Source: CAD feature listing. Evaluate the final solid. Frame: model axes, mm. Coordinates: 2 decimals unless noted, no trailing zeros. Write each loop counter-clockwise with the first axis right and the second up, starting at its lowest first coordinate (ties: lowest second). Pieces come first, ordered by that corner, then holes. Notation, with made-up numbers: (17, 47) -> (30, 47) arc R26 ccw to (30, 66) -> close; hole circle Ø6 at (62.5, 78.25). An arc over 180 degrees is marked (long way). Write item = value, one per line.
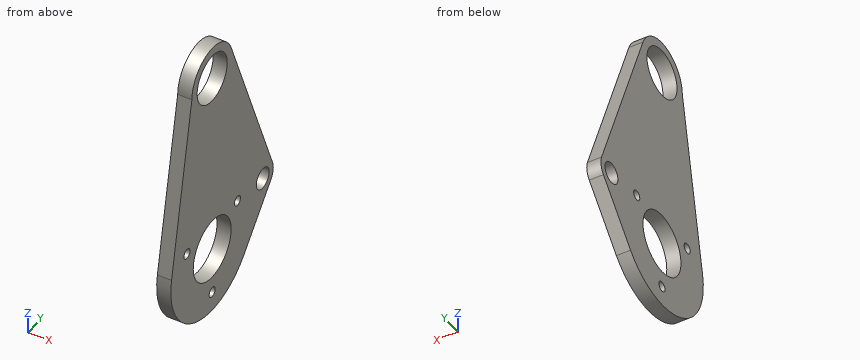
from build123d import *

# Parameters (mm, degrees)
SKETCH1_R            = 11.1125
SKETCH1_R_2          = 14
SKETCH1_R_3          = 4.7625
BOSS_EXTRUDE1_DEPTH  = 3.175
M4_CLEARANCE_HOLE1_D = 4.5


with BuildPart() as part:
    # Sketch1 → Boss-Extrude1 (new, symmetric)
    with BuildSketch(Plane(origin=(0, 0, 0), x_dir=(0, 0, -1), z_dir=(1, 0, 0))):
        with BuildLine():
            ThreePointArc((81.432924752, 43.180446665), (77.696268156, 44.932233649), (73.589867092, 44.521343816))
            Line((73.589867092, 44.521343816), (-5.407259882, 13.991481))
            ThreePointArc((-5.407259882, 13.991481), (-14.745714886, -2.750253171), (0, -15))
            Line((0, -15), (79.344909163, -29.971151924))
            ThreePointArc((79.344909163, -29.971151924), (112.50372992, -13.183127113), (104.821761092, 23.180763301))
            Line((104.821761092, 23.180763301), (81.432924752, 43.180446665))
        make_face()
        Circle(SKETCH1_R, mode=Mode.SUBTRACT)
        with Locations((85, 0)):
            Circle(SKETCH1_R_2, mode=Mode.SUBTRACT)
        with Locations((76.388124081, 37.280752399)):
            Circle(SKETCH1_R_3, mode=Mode.SUBTRACT)
    extrude(amount=BOSS_EXTRUDE1_DEPTH, both=True)

    # M4 Clearance Hole1 (through all)
    with Locations(Plane(origin=(3.175, 0, 0), x_dir=(0, 0, -1), z_dir=(1, 0, 0))):
        with Locations((74.25, 18.619546181), (106.5, 0), (74.25, -18.619546181)):
            Hole(M4_CLEARANCE_HOLE1_D / 2)


solid = part.part
1) Cut plane D-D, the plane y = 39. Output: boundary loops of the cut face in (x, z) (3 decimals), and give its area (3 significant figures).
Answer block:
outline = (-3.175, -86.322) -> (3.175, -86.322) -> (3.175, -80.829) -> (-3.175, -80.829) -> close; (-3.175, -71.947) -> (3.175, -71.947) -> (3.175, -59.303) -> (-3.175, -59.303) -> close
area = 115 mm2
2) First-contact query: pin 1 Ø4 at (y, z) = (18.62, -74.25) entering from +X; pin 2 Ø1.5 at (x, y) = (-1.5, -20.5) entering from -Z. Flat tips, straight axial feed; report the tip coordinate or a pass-through.
Answer block:
pin_1 = through
pin_2 = -108.24
3) Cut plane A-A, the plane z = -106.5. Output: boundary loops of the cut face in (x, y) (3 decimals), and give its area (3 significant figures).
Answer block:
outline = (-3.175, -21.633) -> (3.175, -21.633) -> (3.175, -2.25) -> (-3.175, -2.25) -> close; (-3.175, 2.25) -> (3.175, 2.25) -> (3.175, 21.633) -> (-3.175, 21.633) -> close
area = 246 mm2
4) Material intervals for probe 1 along Y at (x, z) = (1.75, -74.25); probe 2 along Y at (x, z) = (-1.25, -90.5); probe 3 along Y at (x, z) = (0, 0), sorted ascending. Write a range as [from, to].
Answer block:
probe_1 = [-29.01, -20.87], [-16.37, -8.97], [8.97, 16.37], [20.87, 33.03], [41.54, 44.74]
probe_2 = [-30, -12.87], [12.87, 35.43]
probe_3 = [-15, -11.11], [11.11, 16.08]
5) Cut plane C-C, the plane x = 1.5. Give the number of separate pieces and of enclosed holes in the cut face, and give its area (3 significant figures).
Answer block:
separate_pieces = 1
enclosed_holes = 6
area = 5,450 mm2
6) Cut plane B-B, the plane y = -5. Output: boundary loops of the cut face in (x, z) (3 decimals).
Answer block:
outline = (-3.175, -115.087) -> (3.175, -115.087) -> (3.175, -98.077) -> (-3.175, -98.077) -> close; (-3.175, -71.923) -> (3.175, -71.923) -> (3.175, -9.924) -> (-3.175, -9.924) -> close; (-3.175, 9.924) -> (3.175, 9.924) -> (3.175, 14.142) -> (-3.175, 14.142) -> close
